Work out the finished part from the listing and answer in its coordinate system (mm). A direction names the side the tool comes from. Round coordinates to 2 decimals unless told otherwise and drop trailing zeros. Order: outer loops, then holes, each group sorted by start corner. A loop starts at its lowest first (then second) coordinate and runs counter-clockwise, first axis right, second up. Notation, with made-up numbers: (42.5, 85.5) -> (73.5, 85.5) arc R25 ccw to (73.5, 99.5) -> close; hole circle Ø5 at (4.5, -31). An arc over 180 degrees is marked (long way). Use a Markdown table: item, result. Add a question column.
Item 1: A tool of negligible diameter and unlimited length cuts with its end or side. For faces 4 (the cylindrical face through (-6.465, 90.14, -1.035)), 5 (the flat face through (7.5, 30, 0)), 6 (the flat face through (-16, 5, 0.5)), from which of +Z, -Z, +X, -X, +Y, -Y can it reach the whole face along a straight path? Write none if from no direction.
Item 2: A cutting plane is placed at D-D, the plane y = 35. Determine the outline of the cut face in (x, z).
Item 3: Find the intervals of material crossed by L1, parallel to Y at x = 6, z = -1.75; L2, parallel to X at y = 3.5, z = -2.5; L3, parallel to Y at x = 5.5, z = -0.5, in increasing order. Write a range as [from, to].
Item 4: A cutting plane is placed at C-C, the plane x = 9.5. Determine the outline of the cut face in (y, z).
Item 5: A cutting plane is placed at B-B, the plane y = 70. Determine the outline of the cut face in (x, z).
Item 6: Flat-ended cylindrical pins translate along their axes: P1, Ø5.5, axis at x = 0, y = 100, coming from the +Z side; P2, Ø1, axis at y = 74.5, z = 1.5, coming from the -X side; P3, Ø6.5, axis at x = -17.32, y = 70, coming from the -Z side; P4, Ø3, axis at x = 15.5, y = 2.5, coming from the +Z side. Find the tip coordinate at first contact, or state that the pin passes through.
Item 7: A cutting plane is placed at A-A, the plane y = 100. Determine the outline of the cut face in (x, z), plus the area to 3 significant figures.
Item 8: For a pull along X with two mould halves and no side action, classify faces 1 (the flat face through (0, 53, 3.5)), 2 (the cylindrical face through (-16.55, 3.57, -1.53)), 3 (the flat face through (-19, 31, 0)) as +X half, -X half, draft (parallel to the pull), parting line (faces both ways), or undercut.
from build123d import *

# Parameters (mm, degrees)
SKETCH_1_R         = 1.55
SKETCH_1_R_2       = 2.05
SKETCH_1_R_3       = 11
EXTRUDE_1_DEPTH    = 3.5
SKETCH1_R          = 12.025
CUT_EXTRUDE2_DEPTH = 5
SKETCH2_R          = 2.85
CUT_EXTRUDE3_DEPTH = 3
SKETCH3_R          = 3.6
CUT_EXTRUDE4_DEPTH = 4


with BuildPart() as part:
    # 草图1 → 凸台-拉伸1 (new, symmetric)
    with BuildSketch(Plane.XY):
        with BuildLine():
            Line((-19, 0), (19, 0))
            Line((19, 0), (19, 62))
            ThreePointArc((19, 62), (19.25658351, 63.58113883), (20, 65))
            ThreePointArc((20, 65), (0, 105), (-20, 65))
            ThreePointArc((-20, 65), (-19.25658351, 63.58113883), (-19, 62))
            Line((-19, 62), (-19, 0))
        make_face()
        with BuildLine():
            ThreePointArc((-7.5, 45), (0, 52.5), (7.5, 45))
            Line((7.5, 45), (7.5, 15))
            ThreePointArc((7.5, 15), (0, 7.5), (-7.5, 15))
            Line((-7.5, 15), (-7.5, 45))
        make_face(mode=Mode.SUBTRACT)
        with Locations((-15, 3.5)):
            Circle(SKETCH_1_R, mode=Mode.SUBTRACT)
        with Locations((15, 3.5)):
            Circle(SKETCH_1_R, mode=Mode.SUBTRACT)
        with Locations((0, 100)):
            Circle(SKETCH_1_R_2, mode=Mode.SUBTRACT)
        with Locations((-17.320508076, 70)):
            Circle(SKETCH_1_R_2, mode=Mode.SUBTRACT)
        with Locations((0, 80)):
            Circle(SKETCH_1_R_3, mode=Mode.SUBTRACT)
        with Locations((17.320508076, 70)):
            Circle(SKETCH_1_R_2, mode=Mode.SUBTRACT)
    extrude(amount=EXTRUDE_1_DEPTH, both=True)

    # Sketch1 → Cut-Extrude2 (cut)
    with BuildSketch(Plane(origin=(0, 0, -3.5), x_dir=(-1, 0, 0), z_dir=(0, 0, -1))):
        with Locations((0, 80)):
            Circle(SKETCH1_R)
    extrude(amount=-CUT_EXTRUDE2_DEPTH, mode=Mode.SUBTRACT)

    # Sketch2 → Cut-Extrude3 (cut)
    with BuildSketch(Plane.XY.offset(3.5)):
        with Locations((15, 3.5)):
            Circle(SKETCH2_R)
        with Locations(Location((-15, 3.5, 0), (0, 0, 180))):
            Circle(SKETCH2_R)
    extrude(amount=-CUT_EXTRUDE3_DEPTH, mode=Mode.SUBTRACT)

    # Sketch3 → Cut-Extrude4 (cut)
    with BuildSketch(Plane(origin=(0, 0, -3.5), x_dir=(-1, 0, 0), z_dir=(0, 0, -1))):
        with Locations((0, 100)):
            Circle(SKETCH3_R)
        with Locations((17.320508076, 70)):
            Circle(SKETCH3_R)
        with Locations((-17.320508076, 70)):
            Circle(SKETCH3_R)
    extrude(amount=-CUT_EXTRUDE4_DEPTH, mode=Mode.SUBTRACT)


solid = part.part
Reported:
| question | item | result |
|---|---|---|
| 1 | face 4 | -Z |
| 1 | face 5 | +Z, -Z |
| 1 | face 6 | +Z |
| 2 | outline | (-19, -3.5) -> (-7.5, -3.5) -> (-7.5, 3.5) -> (-19, 3.5) -> close; (7.5, -3.5) -> (19, -3.5) -> (19, 3.5) -> (7.5, 3.5) -> close |
| 3 | L1 | [0, 10.5], [49.5, 69.58], [90.42, 104.27] |
| 3 | L2 | [-19, -16.55], [-13.45, 13.45], [16.55, 19] |
| 3 | L3 | [0, 9.9], [50.1, 69.31], [90.69, 104.39] |
| 4 | outline | (0, -3.5) -> (72.63, -3.5) -> (72.63, 1.5) -> (74.45, 1.5) -> (74.45, 3.5) -> (0, 3.5) -> close; (85.55, 1.5) -> (87.37, 1.5) -> (87.37, -3.5) -> (103.12, -3.5) -> (103.12, 3.5) -> (85.55, 3.5) -> close |
| 5 | outline | (-22.91, -3.5) -> (-20.92, -3.5) -> (-20.92, 0.5) -> (-19.37, 0.5) -> (-19.37, 3.5) -> (-22.91, 3.5) -> close; (-15.27, 0.5) -> (-13.72, 0.5) -> (-13.72, -3.5) -> (-6.68, -3.5) -> (-6.68, 1.5) -> (-4.58, 1.5) -> (-4.58, 3.5) -> (-15.27, 3.5) -> close; (4.58, 1.5) -> (6.68, 1.5) -> (6.68, -3.5) -> (13.72, -3.5) -> (13.72, 0.5) -> (15.27, 0.5) -> (15.27, 3.5) -> (4.58, 3.5) -> close; (19.37, 0.5) -> (20.92, 0.5) -> (20.92, -3.5) -> (22.91, -3.5) -> (22.91, 3.5) -> (19.37, 3.5) -> close |
| 6 | P1 | z = 3.5 |
| 6 | P2 | x = -24.49 |
| 6 | P3 | z = 0.5 |
| 6 | P4 | z = 0.5 |
| 7 | outline | (-15, -3.5) -> (-3.6, -3.5) -> (-3.6, 0.5) -> (-2.05, 0.5) -> (-2.05, 3.5) -> (-15, 3.5) -> close; (2.05, 0.5) -> (3.6, 0.5) -> (3.6, -3.5) -> (15, -3.5) -> (15, 3.5) -> (2.05, 3.5) -> close |
| 7 | area | 169 mm² |
| 8 | face 1 | draft |
| 8 | face 2 | undercut |
| 8 | face 3 | -X half |
